Could you check a few things on this model? Use its own coordinates, in mm. Round coordinates to 2 decimals unless told otherwise and drop trailing zeros. Loops run counter-clockwise (first coordinate to the right, second up) from the corner with the lowest first, then second, coordinate; pieces in that order, holes last. Notation, with made-up numbers: (88, -13.75) -> (136, -13.75) arc R22 ccw to (136, 11.25) -> close; hole circle Ø4 at (13.5, 81). An arc over 180 degrees is marked (long way). Write each question's results on one line, items separated by ' | '.
from build123d import *

# Parameters (mm, degrees)
ESQUISSE1_R        = 3
BOSS_EXTRU_1_DEPTH = 33
CHANFREIN1_SIZE    = 0.3


with BuildPart() as part:
    # Esquisse1 → Boss.-Extru.1 (new body)
    with BuildSketch(Plane.XY):
        Circle(ESQUISSE1_R)
    extrude(amount=BOSS_EXTRU_1_DEPTH)

    # Esquisse2 → Enlèvement de matière-Révolution1 (revolve, cut)
    with BuildSketch(Plane(origin=(0, 0, 0), x_dir=(1, 0, 0), z_dir=(0, 1, 0)), mode=Mode.PRIVATE) as enl_vement_de_mati_re_r_volution1_sk:
        Polygon((-10, -2.5), (2, -2.5), (2, -1), (10, -1), (10, -4), (-10, -4), align=None)
    revolve(enl_vement_de_mati_re_r_volution1_sk.sketch.rotate(Axis((10, 0, 4), (1, 0, 0)), 180), axis=Axis((10, 0, 4), (1, 0, 0)), mode=Mode.SUBTRACT)

    # Chanfrein1
    chanfrein1_edges = [part.edges().sort_by_distance(p)[0] for p in [
        (-3, 0, 0),
        (-3, 0, 33),
    ]]
    chamfer(chanfrein1_edges, length=CHANFREIN1_SIZE)


solid = part.part
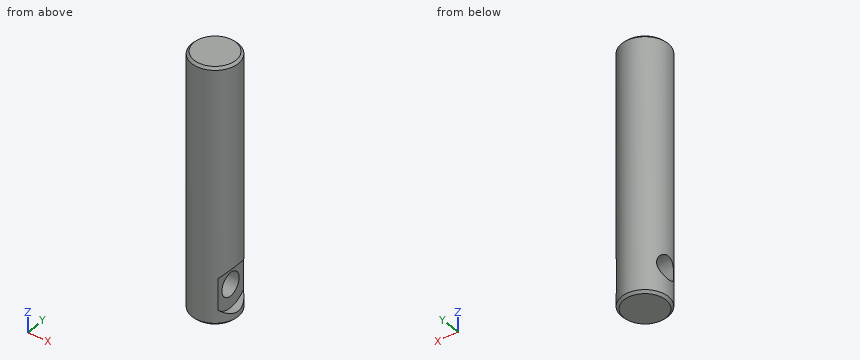
1) I need wall thicknesses on line 1 (Y direction, x = -0.1, z = 4); line 2 (Y direction, x = 0.6, z = 4); line 3 (Z direction, x = -1.5, y = -0.25). Which ranges of each line are inside material? Lowest first, please.
Model answer:
line 1: y = -3 to -1.5, 1.5 to 3 | line 2: y = -2.94 to -1.5, 1.5 to 2.94 | line 3: z = 0 to 2.52, 5.48 to 33
2) I'm going to push a flat-ended pin straight in: pin 1 (2 mm diameter, centred on y = -2, z = 4, fed in from +X). Where does the tip first touch, or does it pass through?
Model answer:
pin 1: stops at x = 2
3) I want a section at C-C, the plane z = 4. Write out the boundary of the cut face in (x, y), plus the area to 3 significant figures.
Model answer:
outline: (-2.6, -1.5) arc R3 ccw to (2, -2.24) -> (2, -1.5) -> close; (-2.6, 1.5) -> (2, 1.5) -> (2, 2.24) arc R3 ccw to start | area: 10.6 mm2
4) I want a section at A-A, the plane y = 0. Write out the boundary of the cut face in (x, z), plus the area to 3 significant figures.
Model answer:
outline: (-3, 0.3) -> (-2.7, 0) -> (2.7, 0) -> (3, 0.3) -> (3, 1) -> (2, 1) -> (2, 2.5) -> (-3, 2.5) -> close; (-3, 5.5) -> (2, 5.5) -> (2, 7) -> (3, 7) -> (3, 32.7) -> (2.7, 33) -> (-2.7, 33) -> (-3, 32.7) -> close | area: 177 mm2
5) I want a section at B-B, the plane x = 0. Write out the boundary of the cut face in (y, z).
Model answer:
outline: (-3, 0.3) -> (-2.7, 0) -> (2.7, 0) -> (3, 0.3) -> (3, 32.7) -> (2.7, 33) -> (-2.7, 33) -> (-3, 32.7) -> close; hole circle Ø3 at (0, 4)
6) I want a section at D-D, the plane z = 14.5. Write out the boundary of the cut face in (x, y), plus the area to 3 significant figures.
Model answer:
outline: circle Ø6 at (0, 0) | area: 28.3 mm2
